```python
from build123d import *

# Parameters (mm, degrees)
BOSS_EXTRUDE1_DEPTH = 25.4
FILLET1_R           = 2.54
SKETCH2_R           = 4.7625
CUT_EXTRUDE1_DEPTH  = 75.818479696


with BuildPart() as part:
    # Sketch1 → Boss-Extrude1 (new body)
    with BuildSketch(Plane.XY):
        with BuildLine():
            Line((0, 32.383567293), (35.8775, 32.383567293))
            ThreePointArc((35.8775, 32.383567293), (43.061704897, 29.40777219), (46.0375, 22.223567293))
            Line((46.0375, 22.223567293), (46.0375, -34.291432707))
            ThreePointArc((46.0375, -34.291432707), (49.757243879, -43.271688828), (58.7375, -46.991432707))
            Line((58.7375, -46.991432707), (79.375, -46.991432707))
            Line((79.375, -46.991432707), (79.375, -40.641432707))
            Line((79.375, -40.641432707), (58.7375, -40.641432707))
            ThreePointArc((58.7375, -40.641432707), (54.247371939, -38.781560767), (52.3875, -34.291432707))
            Line((52.3875, -34.291432707), (52.3875, 22.223567293))
            ThreePointArc((52.3875, 22.223567293), (47.551832957, 33.897900251), (35.8775, 38.733567293))
            Line((35.8775, 38.733567293), (0, 38.733567293))
            Line((0, 38.733567293), (0, 32.383567293))
        make_face()
    extrude(amount=-BOSS_EXTRUDE1_DEPTH)

    # Fillet1
    fillet1_edges = [part.edges().sort_by_distance(p)[0] for p in [
        (79.375, -43.816432707, 0),
        (0, 35.558567293, 0),
        (79.375, -43.816432707, -25.4),
        (0, 35.558567293, -25.4),
    ]]
    fillet(fillet1_edges, radius=FILLET1_R)

    # Sketch2 → Cut-Extrude1 (cut, through all)
    with BuildSketch(Plane(origin=(52.3875, 0, 0), x_dir=(0, 0, -1), z_dir=(1, 0, 0))):
        with Locations(Location((12.7, -15.241432707, 0), (0, 0, 90))):
            Circle(SKETCH2_R)
    extrude(amount=-CUT_EXTRUDE1_DEPTH, mode=Mode.SUBTRACT)


solid = part.part
```
Design review of the part built by this model. Coordinates are the model's own, in mm. A direction names the side the tool comes from. Give positions to 0.01 mm unless a question says otherwise; leave off trailing zeros. Loops run counter-clockwise (first coordinate to the right, second up) from the corner with the lowest first, then second, coordinate; pieces in that order, holes last. Notation, with made-up numbers: M 24.25,86.5 L 60.25,86.5 A10 cw 60.25,102.5 Z; hole C 46,-28.75 d4. An arc over 180 degrees is marked long. Return JSON: item names as keys, results as strings. Group by question number.
Item 1: Insertion check: pin 1 Ø12 at (y, z) = (-24.5, -10) entering from -X; pin 2 Ø5.5 at (y, z) = (-15.24, -12.7) entering from +X; pin 3 Ø12.5 at (y, z) = (-20, -14.5) entering from +X; pin 4 Ø12.5 at (x, z) = (14.5, -6.5) entering from -Y. Each pin has a flat end and moves straight along its axis. Give the tip position at first contact, or say it passes through.
Item 2: Mouldability with a two-part tool opening along Z and no side actions: class faces 1 (the cylindrical face through (49.659, -43.172, -12.522)), 2 (the flat face through (48, 2, -25.4)), 3 (the cylindrical face through (49, -16, -8)), 4 (the cylindrical face through (78.651, -43.772, -0.764)) as released by +Z, released by -Z, zero draft, split by the parting line, or undercut.
Item 3: We need section B-B (x = 66.5). Give the boundary of the cut face in (y, z).
Item 4: We need section C-C (y = -9). Give the boundary of the cut face in (x, z).
Item 5: For probe 1 along Y at (x, z) = (9, -17); probe 2 along X at (y, z) = (-14.5, -3.5); probe 3 along Y at (x, z) = (75, -6.75), list the stretches that pass through material, from the lowest coordinate up.
Item 6: Tool access review of faces 5 (the flat face through (69, -40.641, -13)), 6 (the cylindrical face through (78.651, -43.772, -24.636)), 7 (the flat face through (18, 32.384, -13)): name each direction out of +Z, -Z, +X, -X, +Y, -Y from which nothing blocks a thin tool from reaching the whole face with its end or side.
Output:
{
 "1": {"pin 1": "stops at x = 46.04", "pin 2": "passes through", "pin 3": "stops at x = 52.39", "pin 4": "stops at y = 32.38"},
 "2": {"face 1": "zero draft", "face 2": "released by -Z", "face 3": "undercut", "face 4": "released by +Z"},
 "3": {"outline": "M -46.99,-25.4 L -40.64,-25.4 L -40.64,0 L -46.99,0 Z"},
 "4": {"outline": "M 46.04,-25.4 L 52.39,-25.4 L 52.39,0 L 46.04,0 Z"},
 "5": {"probe 1": "y = 32.38 to 38.73", "probe 2": "x = 46.04 to 52.39", "probe 3": "y = -46.99 to -40.64"},
 "6": {"face 5": "+Z, -Z, +X, +Y", "face 6": "-Z, +X, +Y, -Y", "face 7": "+Z, -Z, -X, -Y"}
}
